Could you check a few things on this model? Use its own coordinates, in mm. A direction names the side the tool comes from. Round coordinates to 2 decimals unless told otherwise and drop trailing zeros. Write each loop counter-clockwise with the first axis right and the second up, starting at its lowest first coordinate (ties: lowest second). Pieces come first, ordered by that corner, then holes. Notation, with made-up numbers: (-15.5, 87) -> (29.5, 87) arc R18 cw to (29.5, 111) -> close; hole circle Ø1 at (49, 36.5). An arc over 180 degrees is marked (long way). Answer in a Markdown table with one row per item. Add a question column.
```python
from build123d import *

# Parameters (mm, degrees)
F0_W     = 50
F0_H     = 235
F1_DEPTH = 4
F2_DEPTH = 10
F3_ANGLE = 180
F5_W     = 50
F5_H     = 5
F6_DEPTH = 32.5


with BuildPart() as f1:
    # F0 (on Top) → F1 (new body)
    with BuildSketch(Plane.XY):
        Rectangle(F0_W, F0_H)
        with BuildLine():
            Line((11, 100), (11, -100))
            ThreePointArc((11, -100), (0, -111), (-11, -100))
            Line((-11, -100), (-11, 100))
            ThreePointArc((-11, 100), (0, 111), (11, 100))
        make_face(mode=Mode.SUBTRACT)
    extrude(amount=F1_DEPTH)

    # F0 (on Top) → F2 (join)
    with BuildSketch(Plane.XY):
        with BuildLine():
            ThreePointArc((-11, -100), (0, -111), (11, -100))
            Line((11, -100), (11, 100))
            ThreePointArc((11, 100), (0, 111), (-11, 100))
            Line((-11, 100), (-11, -100))
        make_face()
        with BuildLine():
            Line((8, 100), (8, -100))
            ThreePointArc((8, -100), (0, -108), (-8, -100))
            Line((-8, -100), (-8, 100))
            ThreePointArc((-8, 100), (0, 108), (8, 100))
        make_face(mode=Mode.SUBTRACT)
    extrude(amount=F2_DEPTH)


with BuildPart() as f1_1:
    # F3: moved
    add(f1.part.rotate(Axis((-8, 0, 0), (0, 1, 0)), F3_ANGLE))


with BuildPart() as f1_2:
    # F4: moved
    add(f1_1.part.moved(Location((16, 0, 0))))

    # F5 (on face) → F6 (join)
    with BuildSketch(Plane.XY):
        with Locations((-0.108881, 114.791463)):
            Rectangle(F5_W, F5_H)
    extrude(amount=F6_DEPTH)


solid = f1_2.part
```
(1) I need wall thicknesses on L1, parallel to Z at x = -12, y = -90.5; L2, parallel to Y at x = -16, z = 22; L3, parallel to Z at x = -10, y = 94.5. Which ranges of each line are inside material? Lowest first, please.
(2) Suppose I cut it at A-A, the plane x = 0. Please give me the cut outline in (y, z), then the cut area to 4 significant figures.
(3) On a 3-axis mill with a long thin cutter (end or side, diameter ignored), from which of +Z, -Z, +X, -X, +Y, -Y can I reach the whole of each face in a straight line? I mean faces 1 (the face through (11, 1, -7)), 2 (the face through (0, 108, -5)), 3 (the face through (0, 112.291, 16)). Say none if no direction works.
(4) Suppose I cut it at B-B, the plane y = 33.5. Please give me the cut outline in (x, z), then the cut area to 3 significant figures.
(5) Suppose I cut it at C-C, the plane x = -17.5. Please give me the cut outline in (y, z), then the cut area to 3 significant figures.
(6) Suppose I cut it at D-D, the plane z = 10. Please give me the cut outline in (x, y).
(7) If we mould it in two halves opening along Y, with no side actions, what happens to faces 4 (the face through (8, -1, -5)), 5 (the face through (11.5, 1.6, -4)), 6 (the face through (0, -117.5, -2))? For each: pulls with the +Y half, pulls with the -Y half, needs draft (parallel to the pull), parting line crosses it, or undercut.
(8) For P1, Ø1, axis at x = 16, z = 23, coming from the -Y side; P2, Ø1.5, axis at y = 23.5, z = -5.5, coming from the -X side; P3, Ø5, axis at y = 11, z = -8, coming from the +X side; P4, Ø6, axis at x = 3.5, y = -74.5, coming from the +Z side, each with a flat end and sliding along its axis, tell me the tip position at first contact or that it passes through.
Response:
| question | item | result |
|---|---|---|
| 1 | L1 | -4 to 0 |
| 1 | L2 | 112.29 to 117.29 |
| 1 | L3 | -10 to 0 |
| 2 | outline | (-117.5, -4) -> (-111, -4) -> (-111, -10) -> (-108, -10) -> (-108, 0) -> (-117.5, 0) -> close; (108, -10) -> (111, -10) -> (111, -4) -> (117.5, -4) -> (117.5, 0) -> (117.29, 0) -> (117.29, 32.5) -> (112.29, 32.5) -> (112.29, 0) -> (108, 0) -> close |
| 2 | area | 274.5 mm² |
| 3 | face 1 | -Z, +X, +Y, -Y |
| 3 | face 2 | +Z, -Z |
| 3 | face 3 | +Z, +X, -X, -Y |
| 4 | outline | (-25, -4) -> (-11, -4) -> (-11, -10) -> (-8, -10) -> (-8, 0) -> (-25, 0) -> close; (8, -10) -> (11, -10) -> (11, -4) -> (25, -4) -> (25, 0) -> (8, 0) -> close |
| 4 | area | 172 mm² |
| 5 | outline | (-117.5, -4) -> (117.5, -4) -> (117.5, 0) -> (117.29, 0) -> (117.29, 32.5) -> (112.29, 32.5) -> (112.29, 0) -> (-117.5, 0) -> close |
| 5 | area | 1,100 mm² |
| 6 | outline | (-25.11, 112.29) -> (24.89, 112.29) -> (24.89, 117.29) -> (-25.11, 117.29) -> close |
| 7 | face 4 | undercut |
| 7 | face 5 | needs draft |
| 7 | face 6 | pulls with the -Y half |
| 8 | P1 | y = 112.29 |
| 8 | P2 | x = -11 |
| 8 | P3 | x = 11 |
| 8 | P4 | through |
